```python
from build123d import *

# Parameters (mm, degrees)
SKETCH1_W                 = 96
SKETCH1_H                 = 96
BOSS_EXTRUDE1_DEPTH       = 8
SKETCH2_W                 = 92
SKETCH2_H                 = 92
COMPONENT_PLATFORM_DEPTH  = 6
CABLE_SLOTS_DEPTH         = 6
SKETCH4_R                 = 7.5
CENTER_MASS_CUT_DEPTH     = 6
INNER_CORNER_FILLETS_R    = 3
SKETCH10_W                = 11
SKETCH10_H                = 10
MOTOR_CUTOUT_DEPTH        = 2
FILLET1_R                 = 3
M3X0_5_TAPPED_HOLE1_D     = 2.5
M3X0_5_TAPPED_HOLE1_DEPTH = 2
F_3_0MM_DOWEL_HOLE1_D     = 3
F_3_0MM_DOWEL_HOLE1_DEPTH = 2
F_3_0MM_DOWEL_HOLE2_D     = 3
F_3_0MM_DOWEL_HOLE2_DEPTH = 2
F_2_0MM_DOWEL_HOLE1_D     = 2
F_2_0MM_DOWEL_HOLE1_DEPTH = 2
F_4_0MM_DOWEL_HOLE1_D     = 4
F_4_0MM_DOWEL_HOLE1_DEPTH = 2
F_3_0MM_DOWEL_HOLE3_D     = 3
F_3_0MM_DOWEL_HOLE3_DEPTH = 2


with BuildPart() as part:
    # Sketch1 → Boss-Extrude1 (new body)
    with BuildSketch(Plane.XY):
        Rectangle(SKETCH1_W, SKETCH1_H)
    extrude(amount=BOSS_EXTRUDE1_DEPTH)

    # Sketch2 → Component Platform (cut)
    with BuildSketch(Plane.XY.offset(8)):
        Rectangle(SKETCH2_W, SKETCH2_H)
    extrude(amount=-COMPONENT_PLATFORM_DEPTH, mode=Mode.SUBTRACT)

    # Sketch3 → Cable Slots (cut, symmetric)
    with BuildSketch(Plane.XY.offset(2)):
        with BuildLine():
            Line((-33.878679656, -25.121320344), (-28.878679656, -20.121320344))
            ThreePointArc((-28.878679656, -20.121320344), (-28.228361402, -19.148050297), (-28, -18))
            Line((-28, -18), (-28, 18))
            ThreePointArc((-28, 18), (-28.228361402, 19.148050297), (-28.878679656, 20.121320344))
            Line((-28.878679656, 20.121320344), (-33.878679656, 25.121320344))
            ThreePointArc((-33.878679656, 25.121320344), (-34.851949703, 25.771638598), (-36, 26))
            Line((-36, 26), (-48, 26))
            Line((-48, 26), (-48, -26))
            Line((-48, -26), (-36, -26))
            ThreePointArc((-36, -26), (-34.851949703, -25.771638598), (-33.878679656, -25.121320344))
        make_face()
        with BuildLine():
            Line((48, -26), (48, 26))
            Line((48, 26), (36, 26))
            ThreePointArc((36, 26), (34.851949703, 25.771638598), (33.878679656, 25.121320344))
            Line((33.878679656, 25.121320344), (28.878679656, 20.121320344))
            ThreePointArc((28.878679656, 20.121320344), (28.228361402, 19.148050297), (28, 18))
            Line((28, 18), (28, -18))
            ThreePointArc((28, -18), (28.228361402, -19.148050297), (28.878679656, -20.121320344))
            Line((28.878679656, -20.121320344), (33.878679656, -25.121320344))
            ThreePointArc((33.878679656, -25.121320344), (34.851949703, -25.771638598), (36, -26))
            Line((36, -26), (48, -26))
        make_face()
    extrude(amount=CABLE_SLOTS_DEPTH, both=True, mode=Mode.SUBTRACT)

    # Sketch4 → Center Mass Cut (cut)
    with BuildSketch(Plane.XY.offset(2)):
        Circle(SKETCH4_R)
    extrude(amount=-CENTER_MASS_CUT_DEPTH, mode=Mode.SUBTRACT)

    # Inner Corner Fillets
    inner_corner_fillets_edges = [part.edges().sort_by_distance(p)[0] for p in [
        (-46, -46, 5),
        (-46, 46, 5),
        (46, 46, 5),
        (46, -46, 5),
    ]]
    fillet(inner_corner_fillets_edges, radius=INNER_CORNER_FILLETS_R)

    # Sketch10 → Motor Cutout (cut)
    with BuildSketch(Plane.XY.offset(2)):
        with Locations((5.5, 0)):
            Rectangle(SKETCH10_W, SKETCH10_H)
    extrude(amount=-MOTOR_CUTOUT_DEPTH, mode=Mode.SUBTRACT)

    # Fillet1
    fillet1_edges = [part.edges().sort_by_distance(p)[0] for p in [
        (11, -5, 1),
        (11, 5, 1),
    ]]
    fillet(fillet1_edges, radius=FILLET1_R)

    # M3x0.5 Tapped Hole1
    with Locations(Plane(origin=(48, 0, 0), x_dir=(0, 0, -1), z_dir=(1, 0, 0))):
        with Locations((-5, -35), (-5, 35)):
            Hole(M3X0_5_TAPPED_HOLE1_D / 2, depth=M3X0_5_TAPPED_HOLE1_DEPTH)

    # Ø3.0mm Dowel Hole1
    with Locations(Plane(origin=(0, 48, 0), x_dir=(1, 0, 0), z_dir=(0, 1, 0))):
        with Locations((35, -5), (-35, -5)):
            f_3_0mm_dowel_hole1 = Hole(F_3_0MM_DOWEL_HOLE1_D / 2, depth=F_3_0MM_DOWEL_HOLE1_DEPTH)

    # Mirror2: Ø3.0mm Dowel Hole1 across plane
    add(f_3_0mm_dowel_hole1.mirror(Plane(origin=(0, 0, 0), x_dir=(0, 0, 1), z_dir=(0, -1, 0))), mode=Mode.SUBTRACT)

    # Ø3.0mm Dowel Hole2
    with Locations(Plane.XY.offset(2)):
        with Locations((-26.5, -26.5), (26.5, -26.5), (26.5, 26.5), (-26.5, 26.5)):
            Hole(F_3_0MM_DOWEL_HOLE2_D / 2, depth=F_3_0MM_DOWEL_HOLE2_DEPTH)

    # Ø2.0mm Dowel Hole1
    with Locations(Plane.XY.offset(2)):
        with Locations((6.72, -6.72), (0, -10), (-6.72, -6.72), (-10, 0), (-6.72, 6.72), (0, 10), (6.72, 6.72)):
            Hole(F_2_0MM_DOWEL_HOLE1_D / 2, depth=F_2_0MM_DOWEL_HOLE1_DEPTH)

    # Ø4.0mm Dowel Hole1
    with Locations(Plane.XY.offset(2)):
        with Locations((-3.74, -20.47), (11.5, -38.25)):
            Hole(F_4_0MM_DOWEL_HOLE1_D / 2, depth=F_4_0MM_DOWEL_HOLE1_DEPTH)

    # Ø3.0mm Dowel Hole3
    with Locations(Plane(origin=(-48, 35, 5), x_dir=(0, 0, -1), z_dir=(-1, 0, 0))):
        with Locations((0, 0), (0, 70)):
            Hole(F_3_0MM_DOWEL_HOLE3_D / 2, depth=F_3_0MM_DOWEL_HOLE3_DEPTH)


solid = part.part
```
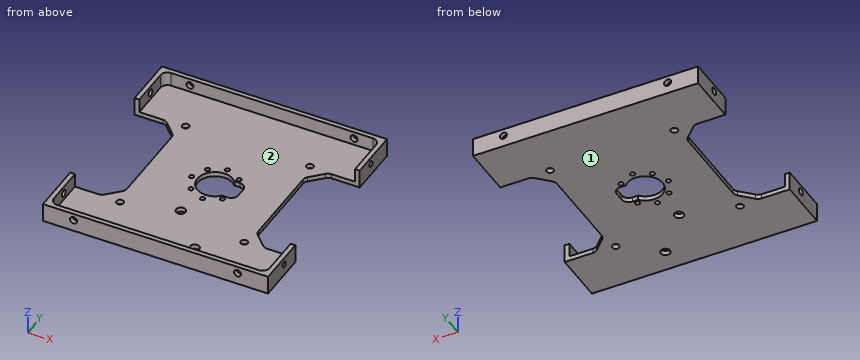
The model under review builds one solid part; all positions refer to its coordinate system, in mm. Face numbers are marked on the shaded views. Round coordinates to 2 decimals unless told otherwise and drop trailing zeros. Loops run counter-clockwise (first coordinate to the right, second up) from the corner with the lowest first, then second, coordinate; pieces in that order, holes last. Notation, with made-up numbers: (41.5, 59.5) - (93.5, 59.5) arc R25 ccw to (93.5, 97.5) - close; hole circle Ø7 at (-17, 51.25). An arc over 180 degrees is marked (long way). Use a Markdown table: item, result. Add a question column.
Q1. Insertion check: pin 1 Ø3 at (y, z) = (23.5, 3) entering from -X; pin 2 Ø1.8 at (x, z) = (-35, 5) entering from +Y; pin 3 Ø2 at (y, z) = (0, 1.5) entering from -X; pin 4 Ø2 at (x, y) = (-22.5, 9.5) entering from +Z. Each pin has a flat end and moves straight along its axis. Give the tip position at first contact, or say it passes through.
Q2. The part is to be moulded in two halves that separate along X. For the marked faces 1 and 2, say which applies: pulls with the +X half, pulls with the -X half, needs draft (parallel to the pull), parting line crosses it, or undercut.
Q3. Add section B-B (x = -3.74). State the section outline as (y, z) points, plus the area to 3 significant figures.
Q4. Add section A-A (y = -38.25). State the section outline as (x, z) points.
Q5. For probe 1 along Y at (x, z) = (-46.8, 5); probe 2 along Y at (x, z) = (6.72, 1.1); probe 3 along Y at (x, z) = (26.5, 1.05), list the stretches that pass through material, from the lowest coordinate up.
Q6. Add section C-C (y = 35). State the section outline as (x, z) points.
Worked answers:
| question | item | result |
|---|---|---|
| 1 | pin 1 | x = -33.38 |
| 1 | pin 2 | through |
| 1 | pin 3 | x = -28 |
| 1 | pin 4 | z = 2 |
| 2 | face 1 | needs draft |
| 2 | face 2 | undercut |
| 3 | outline | (-48, 0) - (-22.47, 0) - (-22.47, 2) - (-46, 2) - (-46, 8) - (-48, 8) - close; (-18.47, 0) - (-6.5, 0) - (-6.5, 2) - (-18.47, 2) - close; (6.5, 0) - (48, 0) - (48, 8) - (46, 8) - (46, 2) - (6.5, 2) - close |
| 3 | area | 182 mm² |
| 4 | outline | (-48, 0) - (9.5, 0) - (9.5, 2) - (-46, 2) - (-46, 8) - (-48, 8) - close; (13.5, 0) - (48, 0) - (48, 8) - (46, 8) - (46, 2) - (13.5, 2) - close |
| 5 | probe 1 | -48 to -36.5, -33.5 to -26, 26 to 33.5, 36.5 to 48 |
| 5 | probe 2 | -48 to -7.72, -5.72 to -5, 5 to 5.72, 7.72 to 48 |
| 5 | probe 3 | -48 to -28, -25 to 25, 28 to 48 |
| 6 | outline | (-48, 0) - (48, 0) - (48, 3.75) - (46, 3.75) - (46, 2) - (-46, 2) - (-46, 3.5) - (-48, 3.5) - close; (-48, 6.5) - (-46, 6.5) - (-46, 8) - (-48, 8) - close; (46, 6.25) - (48, 6.25) - (48, 8) - (46, 8) - close |
